```python
from build123d import *

# Parameters (mm, degrees)
F0_R     = 5
F1_ANGLE = 45
F3_R     = 9.8674102812
F3_R_2   = 5
F2_R     = 5
F4_DEPTH = 10
F6_R     = 9.8674102812
F7_ANGLE = 165
F8_R     = 9.8674102812
F9_ANGLE = 75


# Not quite as in the source:
# - a fillet or chamfer that OpenCascade refuses, or shapes differently, is made with other operations: its cross-section is extruded or revolved along the edge and cut away or added


with BuildPart() as f1:
    # F0 (on Top) → F1 (revolve)
    with BuildSketch(Plane.XY):
        with Locations((17.2625295818, 39.9485491216)):
            Circle(F0_R)
    revolve(axis=Axis((11.3439466804, 38.7977138162, 0), (0, -1, 0)), revolution_arc=F1_ANGLE)

    # F3 (on face) + F2 (on face) → F4 (join)
    with BuildSketch(Plane(origin=(0, 0, 0), x_dir=(1, 0, 0), z_dir=(0, 0, -1))):
        with Locations((17.2625295818, -39.9485491216)):
            Circle(F3_R)
        with Locations((17.2625295818, -39.9485491216)):
            Circle(F3_R_2, mode=Mode.SUBTRACT)
    with BuildSketch(Plane(origin=(0, 0, 0), x_dir=(1, 0, 0), z_dir=(0, 0, -1))):
        with Locations((17.2625295818, -39.9485491216)):
            Circle(F2_R)
    extrude(amount=F4_DEPTH)

    # F5: fillet of radius 5 on 1 edges, made by hand

    # F5_s1 → F5_t2 (revolve, cut)
    with BuildSketch(Plane.XZ.offset(-39.9485491216)):
        with BuildLine():
            ThreePointArc((27.129939863, -4.9982416875), (25.7120445931, -1.5099002903), (22.2625295818, 0))
            Line((22.2625295818, 0), (27.129939863, 0))
            Line((27.129939863, 0), (27.129939863, -4.9982416875))
        make_face()
    revolve(axis=Axis((17.2625295818, 39.9485491216, 0), (0, 0, -1)), mode=Mode.SUBTRACT)

    # F6 (on face) → F7 (revolve)
    with BuildSketch(Plane(origin=(0, 0, -10), x_dir=(1, 0, 0), z_dir=(0, 0, -1))):
        with Locations((17.2625295818, -39.9485491216)):
            Circle(F6_R)
    revolve(axis=Axis((-19.6528339293, 41.1798441783, -10), (0, 1, 0)), revolution_arc=F7_ANGLE)

    # F8 (on face) → F9 (revolve)
    with BuildSketch(Plane(origin=(1.1835097549, 0, -4.4169185366), x_dir=(0.9659258263, 0, 0.2588190451), z_dir=(-0.2588190451, 0, 0.9659258263))):
        with Locations((-58.4867338142, 39.9485491216)):
            Circle(F8_R)
    revolve(axis=Axis((-82.3409964635, 40.3092578053, -26.797242526), (0, -1, 0)), revolution_arc=F9_ANGLE)


solid = f1.part
```
Part model, mm, in its own coordinate system. Coordinates: 2 decimals unless noted, no trailing zeros.
Item 1: Probe line 1 (X direction, y = 48.5, z = -20.5); line 2 (X direction, y = 45.75, z = -14.5); line 3 (Y direction, x = 17.5, z = -2). List the from-to ranges inside material, lowest first.
Item 2: Pin check, flat tips, straight feed: pin 1 (1 mm diameter, centred on y = 35.5, z = -23.5, fed in from +X); pin 2 (6 mm diameter, centred on y = 34, z = -4.5, fed in from +X); pin 3 (3 mm diameter, centred on y = 42.5, z = -6.5, fed in from +X). Stop position of each tip, or through.
Item 3: Mould opens along X. For faces 1 (the face through (9.43, 45.95, -7.46)), 2 (the face through (15.48, 40.019, 4.136)), 3 (the face through (-82.341, 40, 1)) say: released by +X, released by -X, zero draft, split by the parting line, or undercut.
Results found:
1. line 1: x = -60.16 to -49.87, 10.57 to 20.85
1. line 2: x = -66.57 to -48.54, 8.93 to 25.02
1. line 3: y = 31.08 to 48.81
2. pin 1: stops at x = 24.32
2. pin 2: stops at x = 26.67
2. pin 3: stops at x = 27.07
3. face 1: undercut
3. face 2: undercut
3. face 3: released by -X
